Input: part model. Units: mm. Frame: model coordinates. A direction names the side the tool comes from. Coordinates: 2 decimals unless noted, no trailing zeros. Order: outer loops, then holes, each group sorted by start corner. A loop starts at its lowest first (then second) coordinate and runs counter-clockwise, first axis right, second up. Notation, with made-up numbers: (47.25, -24.75) -> (74.25, -24.75) arc R16 cw to (74.25, 5.25) -> close; hole circle Ø6 at (78, 47.5). An arc over 180 degrees is marked (long way). Answer as CSV lines item,"result".
from build123d import *

# Parameters (mm, degrees)
F0_W        = 150.6382748485
F0_H        = 151.164598763
F1_DEPTH    = 76.2
F2_T        = -2.54
F3_T1_DEPTH = 176.0382748485
F4_T1_DEPTH = 158.784598763
F4_T3_DEPTH = 83.82
F4_T6_ANGLE = 89.9999999979
F5_T1_DEPTH = 158.2582748485
F5_T3_DEPTH = 83.82
F5_T6_ANGLE = 89.9999999979
F6_T4_DEPTH = 163.0016440191
F7_W        = 25.6696862793
F7_H        = 42.238175652
F8_DEPTH    = 2.54
F9_W        = 11.248614639
F9_H        = 7.6456852257
F10_DEPTH   = 0.254


# Not quite as in the source:
# - a fillet or chamfer that OpenCascade refuses, or shapes differently, is made with other operations: its cross-section is extruded or revolved along the edge and cut away or added


with BuildPart() as f1:
    # F0 (on Top) → F1 (new body)
    with BuildSketch(Plane.XY):
        with Locations((-0.1240856946, -0.0716410577)):
            Rectangle(F0_W, F0_H)
    extrude(amount=F1_DEPTH)

    # F2
    f2_openings = [f1.faces().sort_by_distance(p)[0] for p in [
        (-0.124086, -0.071641, 76.2),
    ]]
    offset(amount=F2_T, openings=f2_openings)

    # F3: fillet of radius 5.08 on 1 edges, made by hand

    # F3_s2 → F3_t1 (cut)
    with BuildSketch(Plane.YZ.offset(-88.1432231188)):
        with BuildLine():
            ThreePointArc((75.5106583238, 71.12), (74.0227607722, 74.7121024484), (70.4306583238, 76.2))
            Line((70.4306583238, 76.2), (75.5106583238, 76.2))
            Line((75.5106583238, 76.2), (75.5106583238, 71.12))
        make_face()
    extrude(amount=F3_T1_DEPTH, mode=Mode.SUBTRACT)

    # F4: fillet of radius 5.08 on 1 edges, made by hand

    # F4_s2 → F4_t1 (cut)
    with BuildSketch(Plane.XZ.offset(-70.4306583238)):
        with BuildLine():
            ThreePointArc((70.1150517297, 76.2), (73.7071541781, 74.7121024484), (75.1950517297, 71.12))
            Line((75.1950517297, 71.12), (75.1950517297, 76.2))
            Line((75.1950517297, 76.2), (70.1150517297, 76.2))
        make_face()
    extrude(amount=F4_T1_DEPTH, mode=Mode.SUBTRACT)

    # F4_s4 → F4_t3 (cut)
    with BuildSketch(Plane.XY.offset(-12.7)):
        with BuildLine():
            ThreePointArc((70.1150517297, 75.5106583238), (73.7071541781, 74.0227607722), (75.1950517297, 70.4306583238))
            Line((75.1950517297, 70.4306583238), (75.1950517297, 75.5106583238))
            Line((75.1950517297, 75.5106583238), (70.1150517297, 75.5106583238))
        make_face()
    extrude(amount=F4_T3_DEPTH, mode=Mode.SUBTRACT)

    # F4_s5 → F4_t6 (revolve, cut)
    with BuildSketch(Plane.XZ.offset(-70.4306583237)):
        with BuildLine():
            ThreePointArc((70.1150517297, 76.2), (73.7071541781, 74.7121024484), (75.1950517297, 71.12))
            Line((75.1950517297, 71.12), (75.1950517297, 76.2))
            Line((75.1950517297, 76.2), (70.1150517297, 76.2))
        make_face()
    revolve(axis=Axis((75.1950517297, 70.4306583237, 71.1199999999), (-1, 0, 0)), revolution_arc=F4_T6_ANGLE, mode=Mode.SUBTRACT)

    # F5: fillet of radius 5.08 on 1 edges, made by hand

    # F5_s2 → F5_t1 (cut)
    with BuildSketch(Plane.YZ.offset(-88.1432231188)):
        with BuildLine():
            ThreePointArc((-75.6539404392, 71.12), (-74.1660428877, 74.7121024484), (-70.5739404392, 76.2))
            Line((-70.5739404392, 76.2), (-75.6539404392, 76.2))
            Line((-75.6539404392, 76.2), (-75.6539404392, 71.12))
        make_face()
    extrude(amount=F5_T1_DEPTH, mode=Mode.SUBTRACT)

    # F5_s4 → F5_t3 (cut)
    with BuildSketch(Plane.XY.offset(-12.7)):
        with BuildLine():
            ThreePointArc((70.1150517297, -75.6539404392), (73.7071541781, -74.1660428877), (75.1950517297, -70.5739404392))
            Line((75.1950517297, -70.5739404392), (75.1950517297, -75.6539404392))
            Line((75.1950517297, -75.6539404392), (70.1150517297, -75.6539404392))
        make_face()
    extrude(amount=F5_T3_DEPTH, mode=Mode.SUBTRACT)

    # F5_s5 → F5_t6 (revolve, cut)
    with BuildSketch(Plane.YZ.offset(70.1150517296)):
        with BuildLine():
            ThreePointArc((-75.6539404392, 71.12), (-74.1660428877, 74.7121024484), (-70.5739404392, 76.2))
            Line((-70.5739404392, 76.2), (-75.6539404392, 76.2))
            Line((-75.6539404392, 76.2), (-75.6539404392, 71.12))
        make_face()
    revolve(axis=Axis((70.1150517296, -75.6539404392, 71.1199999999), (0, 1, 0)), revolution_arc=F5_T6_ANGLE, mode=Mode.SUBTRACT)

    # F6: fillet of radius 5.08 on 1 edges, made by hand


with BuildPart() as f6_tool2:
    # F6_s3 → F6_t4 (new body)
    with BuildSketch(Plane.XZ.offset(-81.4291809519)):
        with BuildLine():
            ThreePointArc((-75.4432231188, 76.2), (-73.5838140676, 74.3405909488), (-72.9032231188, 71.8005909488))
            Line((-72.9032231188, 71.8005909488), (-72.9032231188, 76.2))
            Line((-72.9032231188, 76.2), (-75.4432231188, 76.2))
        make_face()
    extrude(amount=F6_T4_DEPTH)

    split(bisect_by=Plane.XZ.offset(73.1139404392), keep=Keep.BOTTOM)

    split(bisect_by=Plane.XZ.offset(-72.9706583238), keep=Keep.TOP)


with BuildPart() as f1_1:
    add(f1.part)

    # F6_t1: cut F6_tool2
    add(f6_tool2.part, mode=Mode.SUBTRACT)

    # F7 (on face) → F8 (join)
    with BuildSketch(Plane.XY.offset(2.54)):
        with Locations((-60.0683799791, 51.8515704978)):
            Rectangle(F7_W, F7_H)
    extrude(amount=F8_DEPTH)

    # F9 (on face) → F10 (join)
    with BuildSketch(Plane.XY.offset(5.08)):
        with Locations((-61.2332168967, 65.5658598989)):
            Rectangle(F9_W, F9_H)
    extrude(amount=F10_DEPTH)


solid = f1_1.part
1. Cut plane A-A (z = 31). Return the cut outline in (x, y), plus the area to 3 significant figures.
Findings:
outline,"(-75.44, -75.65) -> (70.12, -75.65) arc R5.08 ccw to (75.2, -70.57) -> (75.2, 70.43) arc R5.08 ccw to (70.12, 75.51) -> (-75.44, 75.51) -> close; hole (-72.9, -73.11) -> (72.66, -73.11) -> (72.66, 72.97) -> (-72.9, 72.97) -> close"
area,"1,500 mm2"
2. Contact query for flat-ended pins moving along their axis: pin 1 (5 mm diameter, centred on x = -22, y = -50.5, fed in from +Z); pin 2 (13 mm diameter, centred on x = -55, y = 61, fed in from +Z). Output: stop coordinate, or through.
Findings:
pin 1,"stops at z = 2.54"
pin 2,"stops at z = 5.33"
3. Mould query, pull axis Y, two halves, no side actions, for faces 1 (the face through (-3.68, 74.62, 73.99)), 2 (the face through (-60, 52, 5.08)), 3 (the face through (-1, 1, 0)), 4 (the face through (-72.903, -1, 37)). Classes: released by +Y, released by -Y, zero draft, split by the parting line, or undercut.
Findings:
face 1,"released by +Y"
face 2,"undercut"
face 3,"zero draft"
face 4,"undercut"
4. Cut plane B-B (y = 48). Return the cut outline in (x, z), plus the area to 3 significant figures.
Findings:
outline,"(-75.44, 0) -> (75.2, 0) -> (75.2, 71.12) arc R5.08 ccw to (72.66, 75.52) -> (72.66, 2.54) -> (-47.23, 2.54) -> (-47.23, 5.08) -> (-72.9, 5.08) -> (-72.9, 71.8) arc R5.08 ccw to (-75.44, 76.2) -> close"
area,"814 mm2"
5. Reachability of faces 5 (the face through (-2, 72.971, 40)), 6 (the face through (74.496, 0.915, 73.692)) from +Z, -Z, +X, -X, +Y, -Y: full face, straight path, thin tool, end or side. Return the list, or none.
Findings:
face 5,"+Z"
face 6,"+Z, +X, +Y, -Y"
6. Ray query, line 1 along X through (y, z) = (28, 43.5); line 2 along Y through (x, z) = (-39, 24.5); line 3 along Z through (x, y) = (-1, -2.5). Return the intervals inside material, ascending.
Findings:
line 1,"x = -75.44 to -72.9, 72.66 to 75.2"
line 2,"y = -75.65 to -73.11, 72.97 to 75.51"
line 3,"z = 0 to 2.54"
7. Cut plane D-D (y = 12). Return the cut outline in (x, z).
Findings:
outline,"(-75.44, 0) -> (75.2, 0) -> (75.2, 71.12) arc R5.08 ccw to (72.66, 75.52) -> (72.66, 2.54) -> (-72.9, 2.54) -> (-72.9, 71.8) arc R5.08 ccw to (-75.44, 76.2) -> close"
8. Cut plane C-C (x = -60.5). Return the cut outline in (y, z).
Findings:
outline,"(-75.65, 0) -> (75.51, 0) -> (75.51, 71.12) arc R5.08 ccw to (72.97, 75.52) -> (72.97, 5.08) -> (69.39, 5.08) -> (69.39, 5.33) -> (61.74, 5.33) -> (61.74, 5.08) -> (30.73, 5.08) -> (30.73, 2.54) -> (-73.11, 2.54) -> (-73.11, 75.52) arc R5.08 ccw to (-75.65, 71.12) -> close"
